Check sheet for the drawn part. Datum: minimum x, y, z corner. Units: mm. Give positions to 0.01 mm unless a question says otherwise; leave off trailing zeros. Order: outer loops, then holes, each group sorted by start corner. A loop starts at its lowest first (then second) coordinate and runs counter-clockwise, first axis right, second up. Notation, with made-up numbers: (18.5, 10.25) -> (67.5, 10.25) arc R14 cw to (67.5, 27.25) -> close; hole circle Ø11 at (-39, -13.75). An arc over 180 degrees is marked (long way). Return JSON: item names as keys, results as strings. Group by question number.
(1) Depth check by flat-ended pin: pin 1 Ø9 at (x, y) = (148, 46) entering from -Z; pin 2 Ø14.5 at (x, y) = (48, 46) entering from +Z. Enter the tip coordinate at first touch or a pass-through.
(2) Cross-section at B-B on y = 200. Enter the section's corners in (x, z), then the cut area to 3 significant figures.
(3) Thickness scan on line 1 along Y through (x, z) = (174, 11); line 2 along Y through (x, z) = (148, 6); line 3 along X through (y, z) = (201, 15.25). Record the ranges inside material, lowest first.
(4) Cross-section at C-C on z = 12. State how many separate pieces and enclosed holes the cut face has, then the cut area to 3 significant figures.
(5) Release check for a two-part mould opening along X. For the marked faces 1 and 2 record: pulls with the +X half, pulls with the -X half, needs draft (parallel to the pull), parting line crosses it, or undercut.
(6) Cross-section at D-D on x = 48. Enter the section's corners in (y, z), then the cut area to 3 significant figures.
(7) Cross-section at A-A on x = 22. Enter the section's corners in (y, z).
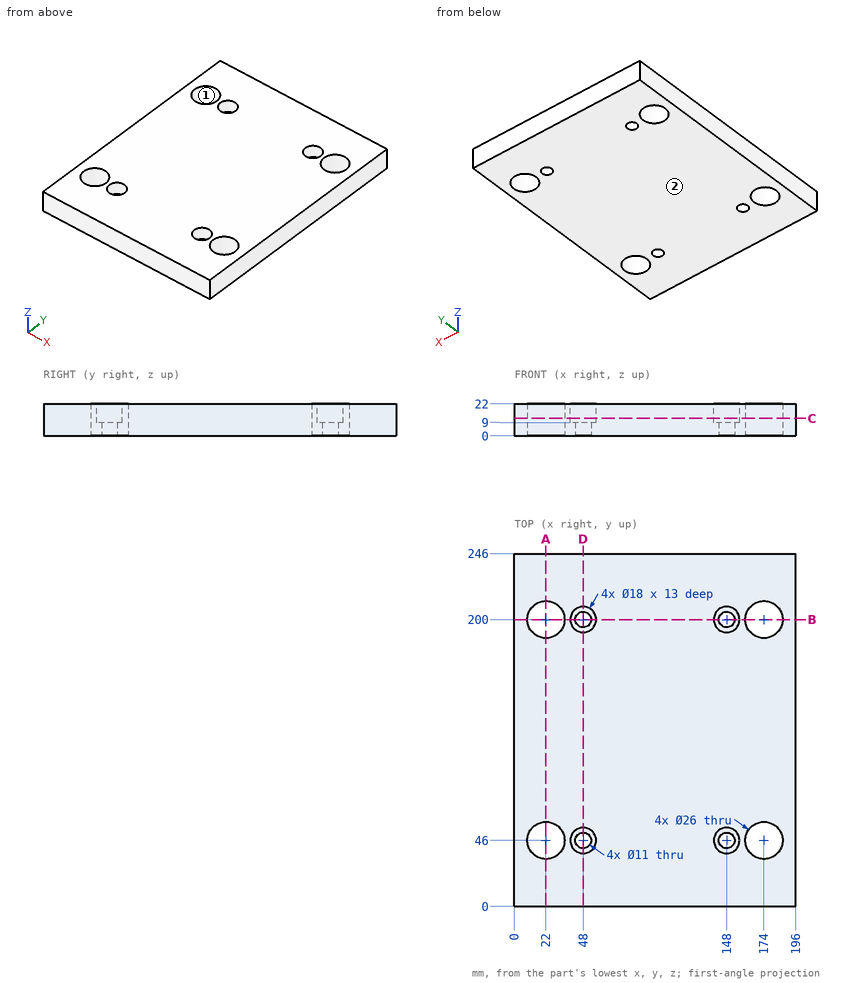
Verdict:
{
 "1": {"pin 1": "through", "pin 2": "z = 9"},
 "2": {"outline": "(0, 0) -> (9, 0) -> (9, 22) -> (0, 22) -> close; (35, 0) -> (42.5, 0) -> (42.5, 9) -> (39, 9) -> (39, 22) -> (35, 22) -> close; (53.5, 0) -> (142.5, 0) -> (142.5, 9) -> (139, 9) -> (139, 22) -> (57, 22) -> (57, 9) -> (53.5, 9) -> close; (153.5, 0) -> (161, 0) -> (161, 22) -> (157, 22) -> (157, 9) -> (153.5, 9) -> close; (187, 0) -> (196, 0) -> (196, 22) -> (187, 22) -> close", "area": "2,500 mm²"},
 "3": {"line 1": "0 to 33, 59 to 187, 213 to 246", "line 2": "0 to 40.5, 51.5 to 194.5, 205.5 to 246", "line 3": "0 to 9.04, 34.96 to 39.06, 56.94 to 139.06, 156.94 to 161.04, 186.96 to 196"},
 "4": {"separate pieces": "1", "enclosed holes": "8", "area": "45,100 mm²"},
 "5": {"face 1": "undercut", "face 2": "needs draft"},
 "6": {"outline": "(0, 0) -> (40.5, 0) -> (40.5, 9) -> (37, 9) -> (37, 22) -> (0, 22) -> close; (51.5, 0) -> (194.5, 0) -> (194.5, 9) -> (191, 9) -> (191, 22) -> (55, 22) -> (55, 9) -> (51.5, 9) -> close; (205.5, 0) -> (246, 0) -> (246, 22) -> (209, 22) -> (209, 9) -> (205.5, 9) -> close", "area": "4,750 mm²"},
 "7": {"outline": "(0, 0) -> (33, 0) -> (33, 22) -> (0, 22) -> close; (59, 0) -> (187, 0) -> (187, 22) -> (59, 22) -> close; (213, 0) -> (246, 0) -> (246, 22) -> (213, 22) -> close"}
}
